Autodesk Inventor part; units mm, degrees
ref_plane "BUFFER_DUMMY_XY" through (0, 0, 0) normal (0, -1, 0) x (1, 0, 0)
ref_plane "BUFFER_DUMMY_YZ" through (0, 0, 0) normal (1, 0, 0) x (0, 0, 1)
ref_plane "BUFFER_DUMMY_ZX" through (0, 0, 0) normal (0, 0, 1) x (0, -1, 0)
sketch "Sketch_9" plane through (0, 0, 0) normal (0, 0, 1) x (1, 0, 0)
  line L0 (0, 12) -> (0, 60)
  line L1 (1.25, 60) -> (1.25, 12)
  line L2 (1.25, 12) -> (2.45, 12)
  line L3 (2.45, 12) -> (2.45, 18)
  line L4 (2.45, 18) -> (3.3865, 18)
  line L5 (3.3865, 18) -> (4, 18.6135)
  line L6 (4, 18.6135) -> (4, 32.3865)
  line L7 (4, 32.3865) -> (3.3865, 33)
  line L8 (3.3865, 33) -> (3.5, 33)
  line L9 (3.5, 33) -> (3.5, 39.35)
  line L10 (3.5, 39.35) -> (4, 39.35)
  line L11 (4, 39.35) -> (6.4, 39.9931)
  line L12 (6.4, 39.9931) -> (6.4, 45.3569)
  line L13 (6.4, 45.3569) -> (4, 46)
  line L14 (4, 46) -> (3.45, 46)
  line L15 (3.45, 46) -> (3.45, 47.3)
  line L16 (3.45, 47.3) -> (3.8105, 47.3)
  line L17 (3.8105, 47.3) -> (6.0968, 47.9126)
  line L18 (6.0968, 47.9126) -> (6.0968, 50.4874)
  line L19 (6.0968, 50.4874) -> (3.8105, 51.1)
  line L20 (3.8105, 51.1) -> (3.95, 51.1)
  line L21 (3.95, 51.1) -> (3.95, 57)
  line L22 (3.95, 57) -> (2.05, 57)
  line L23 (2.05, 57) -> (2.05, 58.5)
  line L24 (2.05, 58.5) -> (4.75, 58.5)
  line L25 (4.75, 58.5) -> (4.75, 60)
  line L26 (4.75, 60) -> (1.25, 60)
revolve "Revolution1" add sketch "Sketch_9" angle 360 about axis through (0, 12, 0) along (0, -1, 0)
thread "Thread1"
sketch "Sketch_10" plane through (0, 51.1, 0) normal (0, 1, 0) x (1, 0, 0)
  circle A0 centre (0, 0) radius 8.8
  line L0 (-4.4, 0) -> (-2.2, -3.8105)
  line L1 (-2.2, -3.8105) -> (2.2, -3.8105)
  line L2 (2.2, -3.8105) -> (4.4, 0)
  line L3 (4.4, 0) -> (2.2, 3.8105)
  line L4 (2.2, 3.8105) -> (-2.2, 3.8105)
  line L5 (-2.2, 3.8105) -> (-4.4, 0)
extrude "Extrusion1" cut sketch "Sketch_10" against normal blind 3.8
sketch "Sketch_11" plane through (0, 46, 0) normal (0, 1, 0) x (1, 0, 0)
  circle A0 centre (0, 0) radius 8
  line L0 (-4.6188, 0) -> (-2.3094, -4)
  line L1 (-2.3094, -4) -> (2.3094, -4)
  line L2 (2.3094, -4) -> (4.6188, 0)
  line L3 (4.6188, 0) -> (2.3094, 4)
  line L4 (2.3094, 4) -> (-2.3094, 4)
  line L5 (-2.3094, 4) -> (-4.6188, 0)
extrude "Extrusion2" cut sketch "Sketch_11" against normal blind 6.65
ref_plane "BUFFER_DUMMY_XY" through (0, 0, 0) normal (0, -1, 0) x (1, 0, 0)
ref_plane "BUFFER_DUMMY_YZ" through (0, 0, 0) normal (1, 0, 0) x (0, 0, 1)
ref_plane "BUFFER_DUMMY_ZX" through (0, 0, 0) normal (0, 0, 1) x (0, -1, 0)
ref_plane "BUFFER_NUT1_XY" through (0, 25.5, 0) normal (0, 1, 0) x (1, 0, 0)
ref_plane "BUFFER_NUT1_YZ" through (0, 25.5, 0) normal (1, 0, 0) x (0, 0, -1)
ref_plane "BUFFER_NUT1_ZX" through (0, 25.5, 0) normal (0, 0, -1) x (0, 1, 0)
ref_plane "BUFFER_NUT2_XY" through (0, 25.5, 0) normal (0, 1, 0) x (1, 0, 0)
ref_plane "BUFFER_NUT2_YZ" through (0, 25.5, 0) normal (1, 0, 0) x (0, 0, -1)
ref_plane "BUFFER_NUT2_ZX" through (0, 25.5, 0) normal (0, 0, -1) x (0, 1, 0)
ref_plane "BUFFER_PLATE_XY" through (0, 25.5, 0) normal (0, 1, 0) x (1, 0, 0)
ref_plane "BUFFER_PLATE_YZ" through (0, 25.5, 0) normal (1, 0, 0) x (0, 0, -1)
ref_plane "BUFFER_PLATE_ZX" through (0, 25.5, 0) normal (0, 0, -1) x (0, 1, 0)
properties part number "ZPT08U6-04_B_BUFFER"
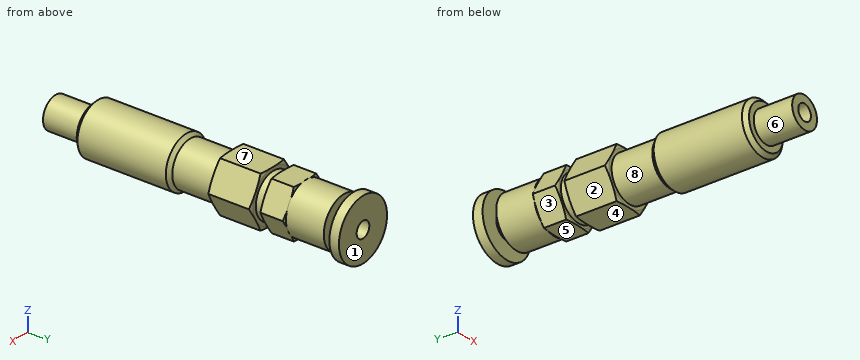
The listing builds one solid part. Answer for the finished solid, in the listing's coordinates (mm). Face numbers are marked on the shaded views. A direction names the side the tool comes from. Give positions to 0.01 mm unless a question says otherwise; leave off trailing zeros. Loops run counter-clockwise (first coordinate to the right, second up) from the corner with the lowest first, then second, coordinate; pieces in that order, holes last. Notation, with made-up numbers: (72, 58.5) - (96, 58.5) arc R19 cw to (96, 71.5) - close; hole circle Ø1 at (64.5, 85). An arc over 180 degrees is marked (long way). Answer as CSV lines item,"result". Start each with the question number.
Item 1: Each of these flat-tipped pins is pushed along its axis until it touches: pin 1 (5 mm diameter, centred on x = -1.5, y = 53, fed in from +Z); pin 2 (3 mm diameter, centred on x = -3.5, y = 22.5, fed in from +Z); pin 3 (4 mm diameter, centred on y = 18.5, z = -3, fed in from +X); pin 4 (2 mm diameter, centred on x = 0, z = 0, fed in from +Y). Where does it stop, or does it pass through?
Item 2: A cutting plane is placed at B-B on y = 43. Determine the outline of the cut face in (x, z).
Item 3: A cutting plane is placed at C-C on y = 29. Determine the outline of the cut face in (x, z), then the cut area to 3 significant figures.
Item 4: A cutting plane is placed at A-A on y = 49. Determine the outline of the cut face in (x, z), then the cut area to 3 significant figures.
Item 5: Find the intervals of material crossed by line 1 (Z direction, x = 0, y = 41.5); line 2 (Z direction, x = 0, y = 34.5); line 3 (Y direction, x = 2.75, z = -1.75), in increasing order. Write a range as from..to.
Item 6: The mould has two halves that part along Y. Classify the marked faces 1, 2 and 3: +Y half, -Y half, draft (parallel to the pull), parting line (faces both ways), or undercut.
Item 7: For the marked faces 4, 5, 6, 7 and 8, determine the directions among +Z, -Z, +X, -X, +Y, -Y from which every point of the face is accessible in a straight line to the end or side of a thin tool.
Found:
1,pin 1,"stops at z = 3.95"
1,pin 2,"stops at z = 3.46"
1,pin 3,"stops at x = 3.87"
1,pin 4,"passes through"
2,outline,"(-4.62, 0) - (-2.31, -4) - (2.31, -4) - (4.62, 0) - (2.31, 4) - (-2.31, 4) - close; hole circle Ø2.5 at (0, 0)"
3,outline,"circle Ø8 at (0, 0); hole circle Ø2.5 at (0, 0)"
3,area,"45.4 mm^2"
4,outline,"(-4.4, 0) - (-2.2, -3.81) - (2.2, -3.81) - (4.4, 0) - (2.2, 3.81) - (-2.2, 3.81) - close; hole circle Ø2.5 at (0, 0)"
4,area,"45.4 mm^2"
5,line 1,"z = -4..-1.25, 1.25..4"
5,line 2,"z = -3.5..-1.25, 1.25..3.5"
5,line 3,"y = 18..57, 58.5..60"
6,face 1,"+Y half"
6,face 2,"draft"
6,face 3,"undercut"
7,face 4,"-Z, +X, -X, -Y"
7,face 5,"-Z, +X, -X"
7,face 6,"-Y"
7,face 7,"+Z, +X, -X, -Y"
7,face 8,"none"
